The model under review builds one solid part; all positions refer to its coordinate system, in mm. Give positions to 0.01 mm unless a question says otherwise; leave off trailing zeros. Order: outer loops, then holes, each group sorted by start corner. A loop starts at its lowest first (then second) coordinate and runs counter-clockwise, first axis right, second up. Notation, with made-up numbers: (83, 84.5) - (124, 84.5) arc R16 ccw to (124, 110.5) - close; hole circle Ø10 at (0, -40). An arc over 180 degrees is marked (long way). Use a Markdown table: item, result. Add a question column.
```python
from build123d import *

# Parameters (mm, degrees)
SKETCH_1_W          = 71
SKETCH_1_H          = 36
EXTRUDE_1_DEPTH     = 47
CUT_EXTRUDE_1_DEPTH = 37
SKETCH_3_R          = 1.5
CUT_EXTRUDE_2_DEPTH = 20


with BuildPart() as part:
    # Эскиз1 → Бобышка-Вытянуть1 (new body)
    with BuildSketch(Plane(origin=(0, 0, 0), x_dir=(1, 0, 0), z_dir=(0, 1, 0))):
        Rectangle(SKETCH_1_W, SKETCH_1_H)
    extrude(amount=EXTRUDE_1_DEPTH)

    # Эскиз2 → Вырез-Вытянуть1 (cut, through all)
    with BuildSketch(Plane.XY.offset(18)):
        Polygon((-20.5, 0), (-35.5, 15), (-35.5, 0), align=None)
        Polygon((35.5, 15), (20.5, 0), (35.5, 0), align=None)
    extrude(amount=-CUT_EXTRUDE_1_DEPTH, mode=Mode.SUBTRACT)

    # Эскиз3 → Вырез-Вытянуть2 (cut)
    with BuildSketch(Plane(origin=(35.5, 0, 0), x_dir=(0, 0, -1), z_dir=(1, 0, 0))):
        with Locations((-7.5, 39)):
            Circle(SKETCH_3_R)
        with Locations((7.5, 39)):
            Circle(SKETCH_3_R)
        with Locations((0, 33)):
            Circle(SKETCH_3_R)
    cut_extrude_2 = extrude(amount=-CUT_EXTRUDE_2_DEPTH, mode=Mode.SUBTRACT)

    # Зеркальное отражение1: Вырез-Вытянуть2 across plane
    add(cut_extrude_2.mirror(Plane(origin=(0, 0, 0), x_dir=(0, 0, 1), z_dir=(1, 0, 0))), mode=Mode.SUBTRACT)


solid = part.part
```
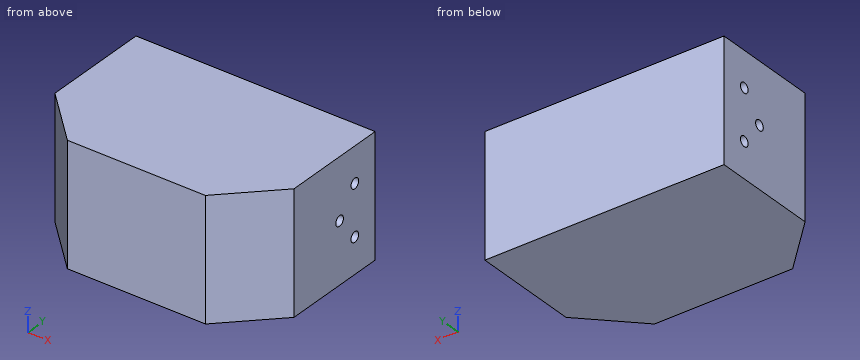
Q1. We need section B-B (y = 39). Write out the cut boundary in (x, z).
Q2. We need section A-A (x = 25.5). Write out the cut boundary in (y, z), plus the area to 3 significant figures.
Q3. Wall thickness on probe 1 along Y at (x, z) = (20.25, 7.5); probe 2 along Y at (x, z) = (29.5, 0); probe 3 along X at (y, z) = (14.5, 2): over which ranges is each line inside the solid? List them lowest first.
Q4. We need section D-D (z = -3.5). Write out the cut boundary in (x, y), plus the area to 3 significant figures.
Q5. Clearance check with flat-ended pins moving along their axes: P1, Ø2.5, axis at y = 39, z = 7.5, coming from the -X side; P2, Ø3.5, axis at y = 39, z = -7.5, coming from the +X side; P3, Ø2.5, axis at y = 33, z = 0, coming from the +X side; P4, Ø1, axis at y = 5.5, z = -6, coming from the +X side. State where each tip first meets the part, or that it passes through.
Q6. We need section C-C (z = -7.5). Write out the cut boundary in (x, y), plus the area to 3 significant figures.
Here are the results:
| question | item | result |
|---|---|---|
| 1 | outline | (-35.5, -18) - (35.5, -18) - (35.5, -9) - (15.5, -9) - (15.5, -6) - (35.5, -6) - (35.5, 6) - (15.5, 6) - (15.5, 9) - (35.5, 9) - (35.5, 18) - (-35.5, 18) - (-35.5, 9) - (-15.5, 9) - (-15.5, 6) - (-35.5, 6) - (-35.5, -6) - (-15.5, -6) - (-15.5, -9) - (-35.5, -9) - close |
| 2 | outline | (5, -18) - (47, -18) - (47, 18) - (5, 18) - close; hole circle Ø3 at (33, 0); hole circle Ø3 at (39, -7.5); hole circle Ø3 at (39, 7.5) |
| 2 | area | 1,490 mm2 |
| 3 | probe 1 | 0 to 37.5, 40.5 to 47 |
| 3 | probe 2 | 9 to 31.5, 34.5 to 47 |
| 3 | probe 3 | -35 to 35 |
| 4 | outline | (-35.5, 15) - (-20.5, 0) - (20.5, 0) - (35.5, 15) - (35.5, 47) - (-35.5, 47) - close |
| 4 | area | 3,110 mm2 |
| 5 | P1 | x = -15.5 |
| 5 | P2 | x = 35.5 |
| 5 | P3 | x = 15.5 |
| 5 | P4 | x = 26.5 |
| 6 | outline | (-35.5, 15) - (-20.5, 0) - (20.5, 0) - (35.5, 15) - (35.5, 37.5) - (15.5, 37.5) - (15.5, 40.5) - (35.5, 40.5) - (35.5, 47) - (-35.5, 47) - (-35.5, 40.5) - (-15.5, 40.5) - (-15.5, 37.5) - (-35.5, 37.5) - close |
| 6 | area | 2,990 mm2 |
